from build123d import *

# Parameters (mm, degrees)
SKETCH_1_W          = 250
SKETCH_1_H          = 100
SKETCH_1_R          = 1.6
EXTRUDE_1_DEPTH     = 4
CUT_EXTRUDE_1_DEPTH = 5


with BuildPart() as part:
    # 草图1 → 凸台-拉伸1 (new body)
    with BuildSketch(Plane(origin=(0, 0, 0), x_dir=(1, 0, 0), z_dir=(0, 1, 0))):
        Rectangle(SKETCH_1_W, SKETCH_1_H)
        with Locations((-115, -40)):
            Circle(SKETCH_1_R, mode=Mode.SUBTRACT)
        with Locations((-85, -40)):
            Circle(SKETCH_1_R, mode=Mode.SUBTRACT)
        with Locations((85, -40)):
            Circle(SKETCH_1_R, mode=Mode.SUBTRACT)
        with Locations((115, -40)):
            Circle(SKETCH_1_R, mode=Mode.SUBTRACT)
    extrude(amount=EXTRUDE_1_DEPTH)

    # 草图2 → 切除-拉伸1 (cut, through all)
    with BuildSketch(Plane(origin=(0, 4, 0), x_dir=(1, 0, 0), z_dir=(0, 1, 0))):
        Polygon((74.999994093, 50), (74.999998028, -10), (-74.999998028, -10), (-74.999994093, 50), align=None)
    extrude(amount=-CUT_EXTRUDE_1_DEPTH, mode=Mode.SUBTRACT)


solid = part.part
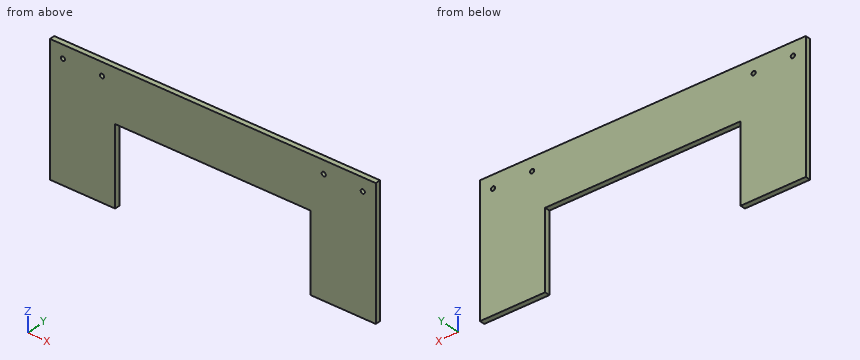
Can you work these out from the model? Positions are in its coordinate system, mm. Give positions to 0.01 mm unless a question says otherwise; leave off trailing zeros. Order: outer loops, then holes, each group sorted by start corner. A loop starts at its lowest first (then second) coordinate and runs counter-clockwise, first axis right, second up. Notation, with made-up numbers: M -26,-24.5 L 14,-24.5 A21 ccw 14,-5.5 Z; hole C 89.5,45 d7. An arc over 180 degrees is marked long. Use a Markdown table: item, result. Add a question column.
Item 1: Suppose I cut it at B-B (y = 2.75). List the corners of the cut face in (x, z) for me.
Item 2: Suppose I cut it at A-A (z = -19). List the corners of the cut face in (x, y) for me, then the cut area to 3 significant figures.
Item 3: If I drill on L1, parallel to X at y = 2.15, z = 40; L2, parallel to Z at x = -115, y = 1.6; L3, parallel to X at y = 1.5, z = 3, over which ranges is the centre line in solid material (lowest first)? Write a range as [from, to].
Item 4: Suppose I cut it at C-C (x = 12). List the corners of the cut face in (y, z) for me.
Item 5: Will these pins go through, and if not, where does the flat tip stop? pin 1 (3 mm diameter, centred on x = 85, z = 40, fed in from +Y); pin 2 (1.2 mm diameter, centred on x = -7, y = 2, fed in from -Z).
Answer sheet:
| question | item | result |
|---|---|---|
| 1 | outline | M -125,-50 L -75,-50 L -75,10 L 75,10 L 75,-50 L 125,-50 L 125,50 L -125,50 Z; hole C -115,40 d3.2; hole C -85,40 d3.2; hole C 85,40 d3.2; hole C 115,40 d3.2 |
| 2 | outline | M -125,0 L -75,0 L -75,4 L -125,4 Z; M 75,0 L 125,0 L 125,4 L 75,4 Z |
| 2 | area | 400 mm² |
| 3 | L1 | x = [-125, -116.6], [-113.4, -86.6], [-83.4, 83.4], [86.6, 113.4], [116.6, 125] |
| 3 | L2 | z = [-50, 38.4], [41.6, 50] |
| 3 | L3 | x = [-125, -75], [75, 125] |
| 4 | outline | M 0,10 L 4,10 L 4,50 L 0,50 Z |
| 5 | pin 1 | passes through |
| 5 | pin 2 | stops at z = 10 |
